from build123d import *

# Parameters (mm, degrees)
BOSS_EXTRU_1_DEPTH           = 15
ENL_V_MAT_EXTRU_2_REACH      = 89.364
ENL_V_MAT_EXTRU_3_REACH      = 88.221
ESQUISSE8_R                  = 5
CHANFREIN1_SIZE              = 0.5
ENL_V_MAT_EXTRU_4_REACH      = 88.221
ENL_V_MAT_EXTRU_4_END_RADIUS = 12.5
ESQUISSE9_R                  = 5
SYM_TRIE2_OUTLINE_R          = 5
SYM_TRIE2_DEPTH              = 5.418281221


# Read off the part's stored shape, not the designer's step: Symétrie2
with BuildPart() as part:
    # Esquisse1 → Boss.-Extru.1 (new body)
    with BuildSketch(Plane.XY):
        with BuildLine():
            Line((-67.384328638, 24.199161074), (-27.384328638, 24.199161074))
            ThreePointArc((-27.384328638, 24.199161074), (-13.384328638, 10.199161074), (-27.384328638, -3.800838926))
            Line((-27.384328638, -3.800838926), (-67.384328638, -3.800838926))
            ThreePointArc((-67.384328638, -3.800838926), (-81.384328638, 10.199161074), (-67.384328638, 24.199161074))
        make_face()
    extrude(amount=BOSS_EXTRU_1_DEPTH)

    # Esquisse3 → Enlèvement de matière-Révolution1 (revolve, cut)
    with BuildSketch(Plane(origin=(0, 10.199161074, 0), x_dir=(-1, 0, 0), z_dir=(0, 1, 0))):
        with BuildLine():
            Line((67.384328638, 28.5), (67.384328638, 3.5))
            ThreePointArc((67.384328638, 3.5), (54.884328638, 16), (67.384328638, 28.5))
        make_face()
    revolve(axis=Axis((-67.384328638, 10.199161074, 28.5), (0, 0, -1)), mode=Mode.SUBTRACT)

    # Esquisse4 → Enlèvement de matière-Révolution2 (revolve, cut)
    with BuildSketch(Plane(origin=(0, 10.199161074, 0), x_dir=(-1, 0, 0), z_dir=(0, 1, 0))):
        with BuildLine():
            Line((27.384328638, 4.374720358), (27.384328638, 29.374720358))
            ThreePointArc((27.384328638, 29.374720358), (39.884328638, 16.874720358), (27.384328638, 4.374720358))
        make_face()
    revolve(axis=Axis((-27.384328638, 10.199161074, 4.374720358), (0, 0, 1)), mode=Mode.SUBTRACT)

    # Esquisse5 → Enlèv. mat.-Extru.2 (cut, up to next)
    with BuildSketch(Plane.XZ.offset(3.800838926), mode=Mode.PRIVATE) as enl_v_mat_extru_2_sk1:
        with BuildLine():
            Line((-63.278251084, 15), (-87.523217527, 15))
            Line((-87.523217527, 15), (-87.523217527, 9))
            Line((-87.523217527, 9), (-68.384328638, 9))
            ThreePointArc((-68.384328638, 9), (-64.141687951, 10.757359313), (-62.384328638, 15))
            Line((-62.384328638, 15), (-63.278251084, 15))
        make_face()
    enl_v_mat_extru_2_tool1 = extrude(enl_v_mat_extru_2_sk1.sketch, amount=-ENL_V_MAT_EXTRU_2_REACH, mode=Mode.PRIVATE) & part.part
    enl_v_mat_extru_2 = enl_v_mat_extru_2_tool1.solids().sort_by_distance((-75.559983, -3.800839, 12.089604))[0]
    add(enl_v_mat_extru_2, mode=Mode.SUBTRACT)

    # Symétrie1: Enlèv. mat.-Extru.2 mirrored; each copy of Enlèv. mat.-Extru.2 runs up to whatever stops it at its own place
    sym_trie1_before = part.part  # the part as the pattern finds it: every copy runs up to it
    sym_trie1_enl_v_mat_extru_2_long = extrude(enl_v_mat_extru_2_sk1.sketch, amount=-ENL_V_MAT_EXTRU_2_REACH, mode=Mode.PRIVATE)
    sym_trie1_enl_v_mat_extru_2_tool1 = sym_trie1_enl_v_mat_extru_2_long.mirror(Plane.ZY.offset(47.384328638)) & sym_trie1_before
    add(sym_trie1_enl_v_mat_extru_2_tool1.solids().sort_by_distance((-19.208674, -3.800839, 12.089604))[0], mode=Mode.SUBTRACT)

    # Esquisse8 → Enlèv. mat.-Extru.3 (cut, up to next)
    with BuildSketch(Plane.XY.offset(15), mode=Mode.PRIVATE) as enl_v_mat_extru_3_sk1:
        with Locations((-47.384328638, 10.199161074)):
            Circle(ESQUISSE8_R)
    enl_v_mat_extru_3_tool1 = extrude(enl_v_mat_extru_3_sk1.sketch, amount=-ENL_V_MAT_EXTRU_3_REACH, mode=Mode.PRIVATE) & part.part
    add(enl_v_mat_extru_3_tool1.solids().sort_by_distance((-47.384329, 10.199161, 15))[0], mode=Mode.SUBTRACT)

    # Chanfrein1
    chanfrein1_edges = [part.edges().sort_by_distance(p)[0] for p in [
        (-52.384328638, 10.199161074, 15),
        (-52.384328638, 10.199161074, 0),
    ]]
    chamfer(chanfrein1_edges, length=CHANFREIN1_SIZE)

    # Enlèv. mat.-Extru.4: up to this sphere (the profile starts outside it)
    enl_v_mat_extru_4_end = Location((-67.384328638, 10.199161074, 16)) * Sphere(ENL_V_MAT_EXTRU_4_END_RADIUS, mode=Mode.PRIVATE)
    # Esquisse9 → Enlèv. mat.-Extru.4 (cut, up to the surface)
    with BuildSketch(Plane(origin=(0, 0, 0), x_dir=(-1, 0, 0), z_dir=(0, 0, -1)), mode=Mode.PRIVATE) as enl_v_mat_extru_4_sk1:
        with Locations((67.384328638, 10.199161074)):
            Circle(ESQUISSE9_R)
    enl_v_mat_extru_4_tool1 = extrude(enl_v_mat_extru_4_sk1.sketch, amount=-ENL_V_MAT_EXTRU_4_REACH, mode=Mode.PRIVATE) - enl_v_mat_extru_4_end
    add(enl_v_mat_extru_4_tool1.solids().sort_by_distance((-67.384329, 10.199161, 0))[0], mode=Mode.SUBTRACT)

    # Symétrie2 outline → Symétrie2 (cut)
    with BuildSketch(Plane.XY):
        with Locations((-27.384328638, 10.199161074)):
            Circle(SYM_TRIE2_OUTLINE_R)
    extrude(amount=SYM_TRIE2_DEPTH, mode=Mode.SUBTRACT)


solid = part.part
The listing builds one solid part. Answer for the finished solid, in the listing's coordinates (mm). A direction names the side the tool comes from. Coordinates: 2 decimals unless noted, no trailing zeros. Order: outer loops, then holes, each group sorted by start corner. A loop starts at its lowest first (then second) coordinate and runs counter-clockwise, first axis right, second up.
Q1. Given P1, Ø9, axis at x = -47.38, y = 10.2, coming from the -Z side; P2, Ø4, axis at x = -25, y = 17.5, coming from the -Z side; P3, Ø1, axis at x = -61.5, y = 17, coming from the +Z side; P4, Ø1.5, axis at y = 9, z = 5.5, coming from the -X side, each flat-ended and moving along its own axis, determine where each tip first touches the part or whether it passes through.
Q2. Consider line 1 (X direction, y = 11, z = 7); line 2 (X direction, y = 14, z = 5.25); line 3 (Y direction, x = -63, z = 2.5). Determine where each line is inside the solid, lowest interval first.
Q3. A cutting plane is placed at B-B, the plane z = 10.5. Write down the section's boundary in (x, y).
Q4. A cutting plane is placed at D-D, the plane y = 18. Write down the section's boundary in (x, z), and give its area (3 significant figures).
Q5. A cutting plane is placed at A-A, the plane x = -65.5. Write down the section's boundary in (y, z).
Q6. A cutting plane is placed at C-C, the plane z = 1.5. Write down the section's boundary in (x, y).
Q7. For a pull along X with two mould halves and no side action, classify faces 3 (the face through (-32.38, 10.42, 2.67)), 4 (the face through (-78, 10, 9)), 5 (the face through (-30.58, 22.48, 10.71)) as pulls with the +X half, pulls with the -X half, needs draft (parallel to the pull), parting line crosses it, or undercut.
Q8. Which of the six approach directions +Z, -Z, +X, -X, +Y, -Y give full straight-line access (tool end or side, diameter ignored) to faces 1 (the face through (-17, 10, 9)), 2 (the face through (-64.2, 22.7, 10.7))?
Answers follow:
1. P1: passes through
1. P2: stops at z = 0
1. P3: stops at z = 7.87
1. P4: stops at x = -81.38
2. line 1: x = -81.36 to -76.02, -58.75 to -52.32, -42.45 to -35.01, -19.76 to -13.41
2. line 2: x = -80.86 to -72.51, -62.26 to -50.63, -44.14 to -30.63, -24.14 to -13.91
2. line 3: y = -3.8 to 7.8, 12.6 to 24.2
3. outline: (-64.42, -3.8) - (-30.35, -3.8) - (-30.35, -0.14) arc R10.75 cw to (-30.35, 20.53) - (-30.35, 24.2) - (-64.42, 24.2) - (-64.42, 21.02) arc R11.22 cw to (-64.42, -0.63) - close; hole circle Ø10 at (-47.38, 10.2)
4. outline: (-79.01, 0) - (-15.76, 0) - (-15.76, 9) - (-21.61, 9) arc R9.77 cw to (-36.97, 15) - (-57.67, 15) arc R9.77 cw to (-74.2, 9) - (-79.01, 9) - close
4. area: 667 mm2
5. outline: (-3.8, 0) - (5.57, 0) - (5.57, 4.54) arc R12.36 cw to (-0.45, 9.74) - (-3.8, 9.74) - close; (14.83, 0) - (24.2, 0) - (24.2, 9.74) - (20.85, 9.74) arc R12.36 cw to (14.83, 4.54) - close
6. outline: (-67.38, -3.8) - (-27.38, -3.8) arc R14 ccw to (-27.38, 24.2) - (-67.38, 24.2) arc R14 ccw to start; hole circle Ø10 at (-67.38, 10.2); hole circle Ø10 at (-47.38, 10.2); hole circle Ø10 at (-27.38, 10.2)
7. face 3: undercut
7. face 4: needs draft
7. face 5: pulls with the +X half
8. face 1: +Z, +X, +Y, -Y
8. face 2: +Z, -X, +Y, -Y
